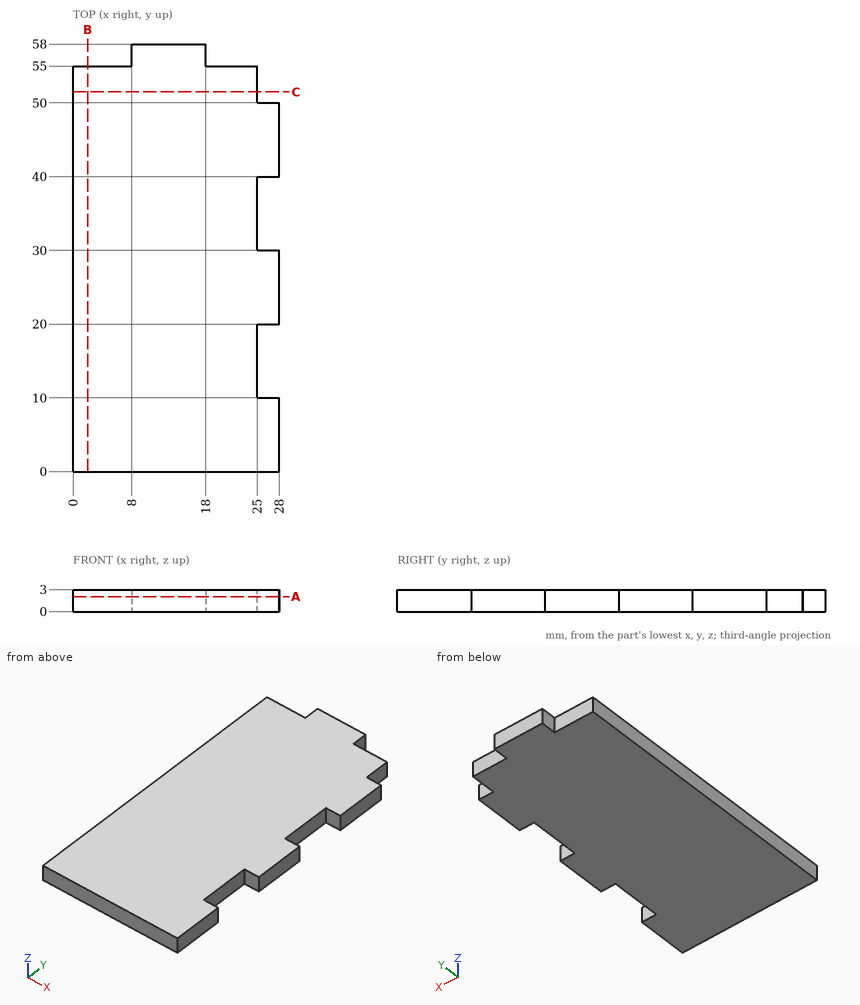
Answer from the drawing. Dimensions are ordinates in mm from the lowest x, y and z of the part. Round coordinates to 2 decimals unless told otherwise and drop trailing zeros. Order: outer loops, then holes, each group sorted by start corner. A loop starts at its lowest first (then second) coordinate and runs counter-clockwise, first axis right, second up.
1) The part is cut by section B-B on x = 2. Write down the section's boundary in (y, z).
2) The part is cut by section C-C on y = 51.5. Write down the section's boundary in (x, z).
3) Flat-ended cylindrical pins translate along their axes: pin 1 (0.9 mm diameter, centred on x = 26.5, z = 1.5, fed in from +Y); pin 2 (1.5 mm diameter, centred on y = 53.5, z = 1, fed in from +X); pin 3 (0.9 mm diameter, centred on y = 56, z = 1, fed in from +X). Find the tip coordinate at first contact, or state that the pin passes through.
4) Straight lines are drawn through the part: L1, parallel to Y at x = 26.5, z = 0.7; L2, parallel to X at y = 15.5, z = 2.4; L3, parallel to Y at x = 24, z = 1.95. For each, find the intervals that lie inside material, in ascending order.
5) The part is cut by section A-A on z = 2.05. Write down the section's boundary in (x, y), plus the area to 4 significant figures.
Resolved:
1. outline: (0, 0) - (55, 0) - (55, 3) - (0, 3) - close
2. outline: (0, 0) - (25, 0) - (25, 3) - (0, 3) - close
3. pin 1: stops at y = 50
3. pin 2: stops at x = 25
3. pin 3: stops at x = 18
4. L1: y = 0 to 10, 20 to 30, 40 to 50
4. L2: x = 0 to 25
4. L3: y = 0 to 55
5. outline: (0, 0) - (28, 0) - (28, 10) - (25, 10) - (25, 20) - (28, 20) - (28, 30) - (25, 30) - (25, 40) - (28, 40) - (28, 50) - (25, 50) - (25, 55) - (18, 55) - (18, 58) - (8, 58) - (8, 55) - (0, 55) - close
5. area: 1,495 mm2
